Input: part model. Units: mm. Frame: model coordinates. Coordinates: 2 decimals unless noted, no trailing zeros. Loops run counter-clockwise (first coordinate to the right, second up) from the corner with the lowest first, then second, coordinate; pieces in that order, holes last. Notation, with made-up numbers: (44.25, 69.5) -> (100.25, 69.5) arc R16 cw to (100.25, 84.5) -> close; hole circle Ø2 at (61.25, 41.25). An arc over 180 degrees is marked (long way). Put each result on its own line as item: value. Start each with the question number.
1) Cut plane B-B (x = -3). Return the cut outline in (y, z).
2) Cut plane C-C (y = 3). Return the cut outline in (x, z), plus the area to 3 significant figures.
3) Material intervals for L1, parallel to Y at x = -11, z = 1.05; L2, parallel to Y at x = 8, z = 3.7; L3, parallel to X at y = -0.5, z = 0.9, sorted ascending.
4) Cut plane A-A (z = 2.1). Return the cut outline in (x, y) (3 decimals), plus the area to 3 significant figures.
from build123d import *

# Parameters (mm, degrees)
F2_DEPTH = 4.15


with BuildPart() as f2:
    # F1 (on Top) → F2 (new body)
    with BuildSketch(Plane.XY):
        with BuildLine():
            ThreePointArc((-0.761124832, -3.3649946494), (-3.45, 0), (-0.761124832, 3.3649946494))
            Line((-0.761124832, 3.3649946494), (-14.55, 1.825))
            ThreePointArc((-14.55, 1.825), (-13.2595301243, 1.2904698757), (-12.725, 0))
            ThreePointArc((-12.725, 0), (-13.2595301243, -1.2904698757), (-14.55, -1.825))
            Line((-14.55, -1.825), (-0.761124832, -3.3649946494))
        make_face()
        with BuildLine():
            ThreePointArc((-12.725, 0), (-13.2595301243, 1.2904698757), (-14.55, 1.825))
            ThreePointArc((-14.55, 1.825), (-16.375, 0), (-14.55, -1.825))
            ThreePointArc((-14.55, -1.825), (-13.2595301243, -1.2904698757), (-12.725, 0))
        make_face()
        with BuildLine():
            ThreePointArc((0.761124832, -3.3649946494), (2.6952161945, -2.1536735279), (3.45, 0))
            ThreePointArc((3.45, 0), (2.6952161945, 2.1536735279), (0.761124832, 3.3649946494))
            Line((0.761124832, 3.3649946494), (0, 3.45))
            Line((0, 3.45), (-0.761124832, 3.3649946494))
            ThreePointArc((-0.761124832, 3.3649946494), (-3.45, 0), (-0.761124832, -3.3649946494))
            Line((-0.761124832, -3.3649946494), (0, -3.45))
            Line((0, -3.45), (0.761124832, -3.3649946494))
        make_face()
        with BuildLine():
            ThreePointArc((0.761124832, 3.3649946494), (2.6952161945, 2.1536735279), (3.45, 0))
            ThreePointArc((3.45, 0), (2.6952161945, -2.1536735279), (0.761124832, -3.3649946494))
            Line((0.761124832, -3.3649946494), (14.55, -1.825))
            ThreePointArc((14.55, -1.825), (12.725, 0), (14.55, 1.825))
            Line((14.55, 1.825), (0.761124832, 3.3649946494))
        make_face()
        with BuildLine():
            ThreePointArc((16.375, 0), (15.8404698757, 1.2904698757), (14.55, 1.825))
            ThreePointArc((14.55, 1.825), (12.725, 0), (14.55, -1.825))
            ThreePointArc((14.55, -1.825), (15.8404698757, -1.2904698757), (16.375, 0))
        make_face()
    extrude(amount=F2_DEPTH)


solid = f2.part
Results found:
1. outline: (-3.11, 0) -> (3.11, 0) -> (3.11, 4.15) -> (-3.11, 4.15) -> close
2. outline: (-4.03, 0) -> (4.03, 0) -> (4.03, 4.15) -> (-4.03, 4.15) -> close
2. area: 33.4 mm2
3. L1: y = -2.22 to 2.22
3. L2: y = -2.56 to 2.56
3. L3: x = -16.31 to 16.31
4. outline: (-14.55, -1.825) -> (0, -3.45) -> (14.55, -1.825) arc R1.825 ccw to (14.55, 1.825) -> (0, 3.45) -> (-14.55, 1.825) arc R1.825 ccw to start
4. area: 164 mm2
